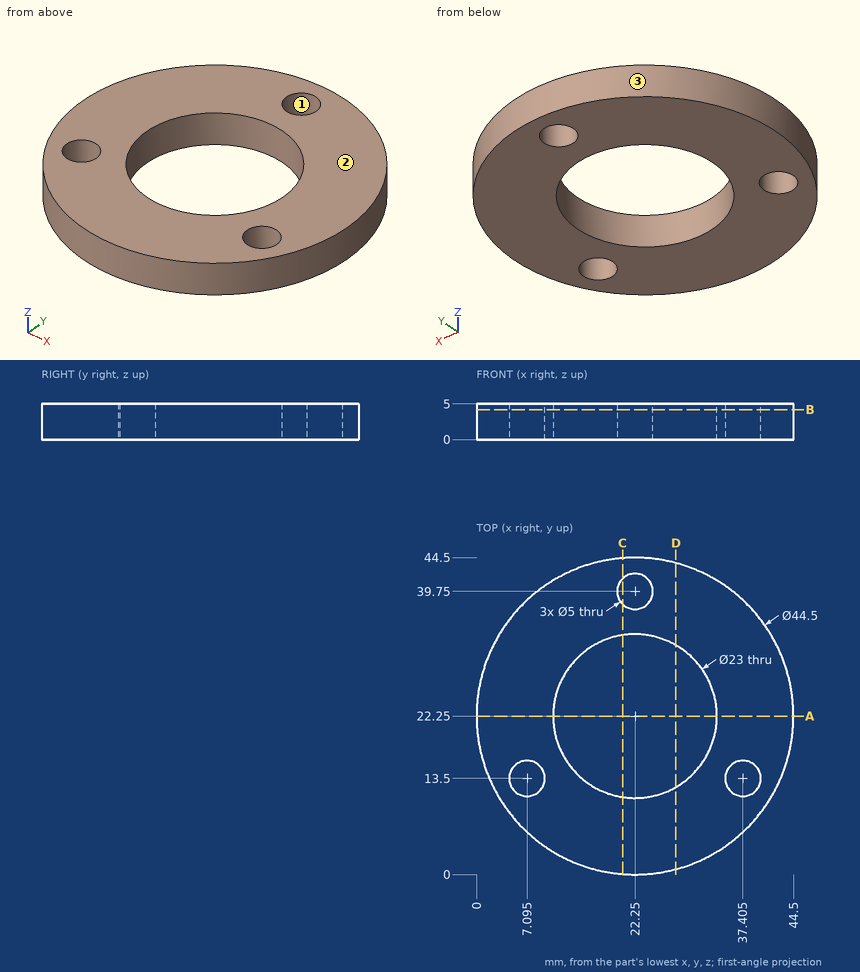
Could you check a few things on this drawing? It's one solid part, dimensions in mm from its lowest x, y, z. Coordinates: 2 decimals unless noted, no trailing zeros. Write each loop counter-clockwise with the first axis right and the second up, starting at its lowest first coordinate (ties: lowest second). Pieces come first, ordered by that corner, then holes.
Q1. Imagine slicing it at D-D, the plane x = 28. List the corners of the cut face in (y, z) for me.
Results found:
outline: (0.76, 0) - (12.29, 0) - (12.29, 5) - (0.76, 5) - close; (32.21, 0) - (43.74, 0) - (43.74, 5) - (32.21, 5) - close
Q2. Imagine slicing it at B-B, the plane z = 4.2. Count the separate pieces of the cut face and the enclosed holes in it, plus the area to 3 significant figures.
Results found:
separate pieces: 1
enclosed holes: 4
area: 1,080 mm2
Q3. Please list where these lines run through material, in increasing order: L1, parallel to Y at x = 22.25, z = 3.15; L2, parallel to X at y = 14, z = 2.6 (1 decimal); L3, parallel to X at y = 31, z = 1.7 (1 decimal).
Results found:
L1: y = 0 to 10.75, 33.75 to 37.25, 42.25 to 44.5
L2: x = 1.6 to 4.6, 9.5 to 14.2, 30.3 to 35, 39.9 to 42.9
L3: x = 1.8 to 14.8, 29.7 to 42.7
Q4. Imagine slicing it at C-C, the plane x = 20.5. List the corners of the cut face in (y, z) for me (1 decimal).
Results found:
outline: (0.1, 0) - (10.9, 0) - (10.9, 5) - (0.1, 5) - close; (33.6, 0) - (38, 0) - (38, 5) - (33.6, 5) - close; (41.5, 0) - (44.4, 0) - (44.4, 5) - (41.5, 5) - close
Q5. For P1, Ø6, axis at x = 22.25, y = 39.75, coming from the -Z side; P2, Ø2, axis at x = 15, z = 4.5, coming from the +Y side; P3, Ø2, axis at y = 38, z = 4.5, coming from the -X side; P4, Ø1.5, axis at x = 14, z = 1.5, coming from the +Y side, each with a flat end and sliding along its axis, tell me the tip position at first contact or that it passes through.
Results found:
P1: stops at z = 0
P2: stops at y = 43.6
P3: stops at x = 5.59
P4: stops at y = 43.2
Q6. If we mould it in two halves opening along Y, with no side actions, what happens to the marked faces 1, 2 and 3? For each: +Y half, -Y half, draft (parallel to the pull), parting line (faces both ways), or undercut.
Results found:
face 1: undercut
face 2: draft
face 3: parting line
Q7. Imagine slicing it at A-A, the plane y = 22.25. List the corners of the cut face in (x, z) for me.
Results found:
outline: (0, 0) - (10.75, 0) - (10.75, 5) - (0, 5) - close; (33.75, 0) - (44.5, 0) - (44.5, 5) - (33.75, 5) - close
